Geometry check sheet. Reference: drawing and pictorial views, mm from the part's lowest x, y, z. A direction names the side the tool comes from. Give positions to 0.01 mm unless a question says otherwise; leave off trailing zeros. Write each loop counter-clockwise with the first axis right and the second up, starting at its lowest first coordinate (ties: lowest second). Pieces come first, ordered by that corner, then holes. Notation, with made-up numbers: (80.25, -3.75) -> (114.25, -3.75) arc R16 ccw to (114.25, 2.25) -> close; hole circle Ø5 at (2, 59.5). An arc over 180 degrees is marked (long way). Use a Markdown table: item, result. Add a question column.
1. Cross-section at C-C (z = 3.5). Enter the section's corners in (x, y) (3 decimals), then the cut area to 3 significant figures.
2. Scan lines: probe 1 along Z at (x, y) = (1.75, 4.5); probe 2 along X at (y, z) = (3.5, 6.25); probe 3 along X at (y, z) = (2.75, 5.25). Record each from-to range of solid material in increasing order. Write a range as [from, to].
3. Cross-section at D-D (x = 2). Enter the section's corners in (y, z), then the cut area to 3 significant figures.
4. Release check for a two-part mould opening along X. For the marked faces 3 and 4 record: released by +X, released by -X, zero draft, split by the parting line, or undercut.
5. Set-up check for the marked faces 1 and 2: record each of +Z, -Z, +X, -X, +Y, -Y from which the full face is reachable in a straight line by a thin tool's end or side.
6. Cross-section at B-B (x = 3.25). Enter the section's corners in (y, z).
7. Gauge pin test, flat ends, axial feed: P1, Ø1, axis at y = 4, z = 10, coming from the -X side; P2, Ø2, axis at y = 4, z = 13.5, coming from the +X side; P3, Ø2, axis at y = 5, z = 11.5, coming from the +X side. Record the tip position at first contact, or that the pin passes through.
8. Cross-section at A-A (y = 4). Enter the section's corners in (x, z), then the cut area to 3 significant figures.
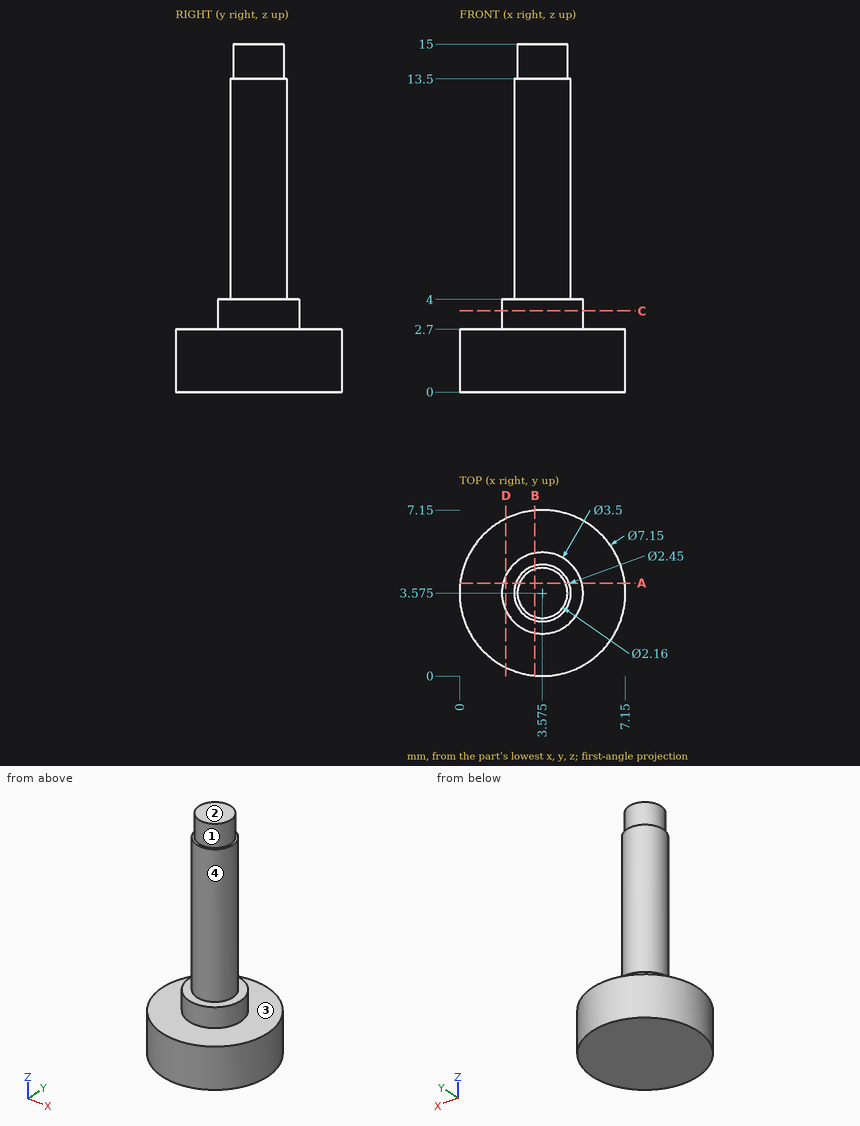
Worked answers:
| question | item | result |
|---|---|---|
| 1 | outline | circle Ø3.5 at (3.575, 3.575) |
| 1 | area | 9.62 mm² |
| 2 | probe 1 | z = [0, 2.7] |
| 2 | probe 2 | x = [2.35, 4.8] |
| 2 | probe 3 | x = [2.67, 4.48] |
| 3 | outline | (0.37, 0) -> (6.78, 0) -> (6.78, 2.7) -> (4.34, 2.7) -> (4.34, 4) -> (2.81, 4) -> (2.81, 2.7) -> (0.37, 2.7) -> close |
| 3 | area | 19.3 mm² |
| 4 | face 3 | zero draft |
| 4 | face 4 | split by the parting line |
| 5 | face 1 | +Z |
| 5 | face 2 | +Z, +X, -X, +Y, -Y |
| 6 | outline | (0.01, 0) -> (7.14, 0) -> (7.14, 2.7) -> (5.29, 2.7) -> (5.29, 4) -> (4.76, 4) -> (4.76, 13.5) -> (4.6, 13.5) -> (4.6, 15) -> (2.55, 15) -> (2.55, 13.5) -> (2.39, 13.5) -> (2.39, 4) -> (1.86, 4) -> (1.86, 2.7) -> (0.01, 2.7) -> close |
| 7 | P1 | stops at x = 2.35 |
| 7 | P2 | stops at x = 4.8 |
| 7 | P3 | stops at x = 4.72 |
| 8 | outline | (0.03, 0) -> (7.12, 0) -> (7.12, 2.7) -> (5.27, 2.7) -> (5.27, 4) -> (4.72, 4) -> (4.72, 13.5) -> (4.57, 13.5) -> (4.57, 15) -> (2.58, 15) -> (2.58, 13.5) -> (2.43, 13.5) -> (2.43, 4) -> (1.88, 4) -> (1.88, 2.7) -> (0.03, 2.7) -> close |
| 8 | area | 48.4 mm² |
